```python
from build123d import *

# Parameters (mm, degrees)
SKETCH1_R           = 1.5
BOSS_EXTRUDE1_DEPTH = 6.9
CUT_EXTRUDE2_DEPTH  = 4.9
SKETCH5_R           = 1
CUT_EXTRUDE3_DEPTH  = 7
SKETCH8_R           = 1
CUT_EXTRUDE5_DEPTH  = 17


with BuildPart() as part:
    # Sketch1 → Boss-Extrude1 (new body)
    with BuildSketch(Plane.XY):
        with BuildLine():
            Line((0, 0), (0, 18.000341084))
            Line((0, 18.000341084), (4, 18.000341084))
            Line((4, 18.000341084), (4, 14.000341084))
            Line((4, 14.000341084), (9.631516349, 14.000341084))
            Line((9.631516349, 14.000341084), (9.631516349, 18.000341084))
            Line((9.631516349, 18.000341084), (31.10792826, 13.336453737))
            ThreePointArc((31.10792826, 13.336453737), (36.383041872, 6.025227564), (29.676516349, 0))
            Line((29.676516349, 0), (9.631516349, 0))
            Line((9.631516349, 0), (9.631516349, 4))
            Line((9.631516349, 4), (4, 4))
            Line((4, 4), (4, 0))
            Line((4, 0), (0, 0))
        make_face()
        with Locations((29.676516349, 6.745044143)):
            Circle(SKETCH1_R, mode=Mode.SUBTRACT)
    extrude(amount=BOSS_EXTRUDE1_DEPTH)

    # Sketch4 → Cut-Extrude2 (cut)
    with BuildSketch(Plane.XY):
        with BuildLine():
            Line((21.876472206, 0), (21.876472206, 15.341186709))
            Line((21.876472206, 15.341186709), (31.10792826, 13.336453737))
            ThreePointArc((31.10792826, 13.336453737), (36.383041872, 6.025227564), (29.676516349, 0))
            Line((29.676516349, 0), (21.876472206, 0))
        make_face()
    extrude(amount=CUT_EXTRUDE2_DEPTH, mode=Mode.SUBTRACT)

    # Sketch5 → Cut-Extrude3 (cut)
    with BuildSketch(Plane.ZY):
        with Locations((2.45, 8)):
            Circle(SKETCH5_R)
    extrude(amount=-CUT_EXTRUDE3_DEPTH, mode=Mode.SUBTRACT)

    # Sketch8 → Cut-Extrude5 (cut)
    with BuildSketch(Plane(origin=(24.246323118, 6.496782699, 0), x_dir=(0, 0, -1), z_dir=(0.965925826, 0.258819045, 0))):
        with Locations((-2.45, 6.201190468)):
            Circle(SKETCH8_R)
    extrude(amount=-CUT_EXTRUDE5_DEPTH, mode=Mode.SUBTRACT)


solid = part.part
```
Work out the finished part from the listing and answer in its coordinate system (mm). A direction names the side the tool comes from. Round coordinates to 2 decimals unless told otherwise and drop trailing zeros. Write each loop counter-clockwise with the first axis right and the second up, starting at its lowest first coordinate (ties: lowest second). Pieces come first, ordered by that corner, then holes. Notation, with made-up numbers: (32.25, -6) -> (46.25, -6) arc R23 cw to (46.25, 5) -> close; hole circle Ø5 at (39.5, -3). An arc over 180 degrees is marked (long way). Write each question's results on one line, items separated by ' | '.
Q1. Section D-D, the plane z = 5.5 is taken. Write down the section's boundary in (x, y), then the cut area to 3 significant figures.
Data:
outline: (0, 0) -> (4, 0) -> (4, 4) -> (9.63, 4) -> (9.63, 0) -> (29.68, 0) arc R6.75 ccw to (31.11, 13.34) -> (9.63, 18) -> (9.63, 14) -> (4, 14) -> (4, 18) -> (0, 18) -> close; hole circle Ø3 at (29.68, 6.75) | area: 510 mm^2
Q2. Section A-A, the plane z = 2.45 is taken. Write down the section's boundary in (x, y), then the cut area to 3 significant figures.
Data:
outline: (0, 0) -> (4, 0) -> (4, 4) -> (9.63, 4) -> (9.63, 0) -> (21.88, 0) -> (21.88, 11.25) -> (7, 7.26) -> (7, 7) -> (0, 7) -> close; (0, 9) -> (5.98, 9) -> (5.96, 9.05) -> (21.88, 13.32) -> (21.88, 15.34) -> (9.63, 18) -> (9.63, 14) -> (4, 14) -> (4, 18) -> (0, 18) -> close | area: 287 mm^2
Q3. Section C-C, the plane x = 29 is taken. Write down the section's boundary in (y, z), then the cut area to 3 significant figures.
Data:
outline: (0, 4.9) -> (5.41, 4.9) -> (5.41, 6.9) -> (0, 6.9) -> close; (8.08, 4.9) -> (13.79, 4.9) -> (13.79, 6.9) -> (8.08, 6.9) -> close | area: 22.2 mm^2
Q4. Determine the mould class of faces 1 (the flat face through (18, 0, 4)), 2 (the flat face through (7, 14, 3)), 3 (the flat face through (17.83, 16.22, 4.17)), 4 (the flat face through (9.632, 16, 3)) for opening direction X: released by +X, released by -X, zero draft, split by the parting line, or undercut.
Data:
face 1: zero draft | face 2: undercut | face 3: released by +X | face 4: undercut
Q5. Section B-B, the plane y = 6.25 is taken. Write down the section's boundary in (x, z).
Data:
outline: (0, 0) -> (21.88, 0) -> (21.88, 4.9) -> (28.26, 4.9) -> (28.26, 6.9) -> (0, 6.9) -> close; (31.09, 4.9) -> (36.4, 4.9) -> (36.4, 6.9) -> (31.09, 6.9) -> close
Q6. Flat-ended cylindrical pins translate along their axes: P1, Ø3, axis at x = 8, z = 2, coming from the -Y side; P2, Ø3, axis at x = 17, z = 2, coming from the -Y side; P3, Ø1.8, axis at y = 8, z = 2.45, coming from the -X side; P4, Ø1.7, axis at x = 6, z = 3, coming from the +Y side. Find the tip coordinate at first contact, or state that the pin passes through.
Data:
P1: y = 4 | P2: y = 0 | P3: x = 7 | P4: y = 14
Q7. Straight lines are drawn through the part: line 1 along X through (y, z) = (3, 1.5); line 2 along Y through (x, z) = (2, 2.45); line 3 along Y through (x, z) = (4.25, 2.45). For each, find the intervals that lie inside material, in ascending order. Write a range as [from, to].
Data:
line 1: [0, 4], [9.63, 21.88] | line 2: [0, 7], [9, 18] | line 3: [4, 7], [9, 14]
Q8. Which of the six approach directions +Z, -Z, +X, -X, +Y, -Y give full straight-line access (tool end or side, diameter ignored) to faces 5 (the cylindrical face through (3.451, 7.024, 2.233)), 6 (the flat face through (7, 4, 3)), 7 (the flat face through (28, 8, 4.9)), 8 (the flat face through (4, 16, 3))?
Data:
face 5: -X | face 6: +Z, -Z, -Y | face 7: -Z, +X, +Y, -Y | face 8: +Z, -Z, +Y
